Model file for the job. Use its own axes, mm. A direction names the side the tool comes from. Give positions to 0.01 mm unless a question says otherwise; leave off trailing zeros. Order: outer loops, then holes, each group sorted by start corner. A loop starts at its lowest first (then second) coordinate and runs counter-clockwise, first axis right, second up. Notation, with made-up numbers: M 55.5,-38 L 108.5,-38 A21 cw 108.5,-27 Z; hole C -34,6 d5. An arc over 180 degrees is marked long. Return JSON: item names as keys, results as strings. Group by question number.
1. Two-plate mould, pull along Y, no slides. Class faces 1 (the face through (0, 6, 0)), 2 (the face through (10, 3, 0)), 3 (the face through (-2.5, 22, -23)): released by +Y, released by -Y, zero draft, split by the parting line, or undercut.
2. Slice it at B-B on y = 22.5. List the corners of the cut face in (x, z).
3. Slice it at D-D on y = 5. List the corners of the cut face in (x, z).
4. Slice it at A-A on x = -20. List the corners of the cut face in (y, z).
5. Slice it at C-C on z = -8.5. List the corners of the cut face in (x, y).
6. Wall check: probe 1 along X at (y, z) = (23, -22.5); probe 2 along X at (y, z) = (32.5, -5); probe 3 along Y at (x, z) = (-5.5, -7.5). Give the ranges that are in metal, low to high. Write a range as [from, to].
7. 3-axis set-ups, long thin cutter, end or side, ignore diameter. For faces 4 (the face through (-2.5, 22, 22)), 5 (the face through (0, 17, 25)), 6 (the face through (-2.5, 5, -23)), 7 (the face through (22, 5, 2.5)), 8 (the face through (-22, 5, 2.5)): which of +Z, -Z, +X, -X, +Y, -Y reach the whole face in a straight line?
from build123d import *

# Parameters (mm, degrees)
SKETCH1_W           = 50
SKETCH1_H           = 50
BOSS_EXTRUDE1_DEPTH = 35
SKETCH3_W           = 5
SKETCH3_H           = 5
CUT_EXTRUDE2_DEPTH  = 6
SKETCH4_W           = 5
SKETCH4_H           = 5
CUT_EXTRUDE3_DEPTH  = 5
SKETCH5_W           = 5
SKETCH5_H           = 5
CUT_EXTRUDE4_DEPTH  = 6
SKETCH6_W           = 5
SKETCH6_H           = 5
CUT_EXTRUDE5_DEPTH  = 6
SKETCH7_W           = 20
SKETCH7_H           = 20
CUT_EXTRUDE6_DEPTH  = 6
SKETCH8_W           = 20
SKETCH8_H           = 20
CUT_EXTRUDE7_DEPTH  = 6


with BuildPart() as part:
    # Sketch1 → Boss-Extrude1 (new body)
    with BuildSketch(Plane(origin=(0, 0, 0), x_dir=(1, 0, 0), z_dir=(0, 1, 0))):
        Rectangle(SKETCH1_W, SKETCH1_H)
    extrude(amount=BOSS_EXTRUDE1_DEPTH)

    # Sketch3 → Cut-Extrude2 (cut)
    with BuildSketch(Plane.ZY.offset(25)):
        with Locations((0, 5)):
            Rectangle(SKETCH3_W, SKETCH3_H)
        with Locations((0, 22.5)):
            Rectangle(SKETCH3_W, SKETCH3_H)
    extrude(amount=-CUT_EXTRUDE2_DEPTH, mode=Mode.SUBTRACT)

    # Sketch4 → Cut-Extrude3 (cut)
    with BuildSketch(Plane(origin=(0, 0, -25), x_dir=(-1, 0, 0), z_dir=(0, 0, -1))):
        with Locations((0, 5)):
            Rectangle(SKETCH4_W, SKETCH4_H)
        with Locations((0, 22.5)):
            Rectangle(SKETCH4_W, SKETCH4_H)
    extrude(amount=-CUT_EXTRUDE3_DEPTH, mode=Mode.SUBTRACT)

    # Sketch5 → Cut-Extrude4 (cut)
    with BuildSketch(Plane(origin=(25, 0, 0), x_dir=(0, 0, -1), z_dir=(1, 0, 0))):
        with Locations((0, 5)):
            Rectangle(SKETCH5_W, SKETCH5_H)
        with Locations((0, 22.5)):
            Rectangle(SKETCH5_W, SKETCH5_H)
    extrude(amount=-CUT_EXTRUDE4_DEPTH, mode=Mode.SUBTRACT)

    # Sketch6 → Cut-Extrude5 (cut)
    with BuildSketch(Plane.XY.offset(25)):
        with Locations((0, 5)):
            Rectangle(SKETCH6_W, SKETCH6_H)
        with Locations((0, 22.5)):
            Rectangle(SKETCH6_W, SKETCH6_H)
    extrude(amount=-CUT_EXTRUDE5_DEPTH, mode=Mode.SUBTRACT)

    # Sketch7 → Cut-Extrude6 (cut)
    with BuildSketch(Plane(origin=(0, 0, 0), x_dir=(-1, 0, 0), z_dir=(0, -1, 0))):
        Rectangle(SKETCH7_W, SKETCH7_H)
    extrude(amount=-CUT_EXTRUDE6_DEPTH, mode=Mode.SUBTRACT)

    # Sketch8 → Cut-Extrude7 (cut)
    with BuildSketch(Plane(origin=(0, 35, 0), x_dir=(1, 0, 0), z_dir=(0, 1, 0))):
        Rectangle(SKETCH8_W, SKETCH8_H)
    extrude(amount=-CUT_EXTRUDE7_DEPTH, mode=Mode.SUBTRACT)


solid = part.part
Result:
{
 "1": {"face 1": "released by -Y", "face 2": "zero draft", "face 3": "undercut"},
 "2": {"outline": "M -25,-25 L -2.5,-25 L -2.5,-20 L 2.5,-20 L 2.5,-25 L 25,-25 L 25,-2.5 L 19,-2.5 L 19,2.5 L 25,2.5 L 25,25 L 2.5,25 L 2.5,19 L -2.5,19 L -2.5,25 L -25,25 L -25,2.5 L -19,2.5 L -19,-2.5 L -25,-2.5 Z"},
 "3": {"outline": "M -25,-25 L -2.5,-25 L -2.5,-20 L 2.5,-20 L 2.5,-25 L 25,-25 L 25,-2.5 L 19,-2.5 L 19,2.5 L 25,2.5 L 25,25 L 2.5,25 L 2.5,19 L -2.5,19 L -2.5,25 L -25,25 L -25,2.5 L -19,2.5 L -19,-2.5 L -25,-2.5 Z; hole M -10,-10 L 10,-10 L 10,10 L -10,10 Z"},
 "4": {"outline": "M 0,-25 L 35,-25 L 35,25 L 0,25 Z; hole M 2.5,-2.5 L 7.5,-2.5 L 7.5,2.5 L 2.5,2.5 Z; hole M 20,-2.5 L 25,-2.5 L 25,2.5 L 20,2.5 Z"},
 "5": {"outline": "M -25,0 L -10,0 L -10,6 L 10,6 L 10,0 L 25,0 L 25,35 L 10,35 L 10,29 L -10,29 L -10,35 L -25,35 Z"},
 "6": {"probe 1": "x = [-25, -2.5], [2.5, 25]", "probe 2": "x = [-25, -10], [10, 25]", "probe 3": "y = [6, 29]"},
 "7": {"face 4": "+Z", "face 5": "+Z, +X, -X, +Y, -Y", "face 6": "-Z", "face 7": "+X", "face 8": "-X"}
}
